```python
from build123d import *

# Parameters (mm, degrees)
F0_R      = 13
F5_DEPTH  = 15
F4_R      = 8
F6_DEPTH  = 15
F3_R      = 3.2
F8_DEPTH  = 4
F9_DEPTH  = 11
F10_R     = 2.05
F11_DEPTH = 15
F12_R     = 1.5
F13_DEPTH = 25
F15_R     = 3.5
F16_DEPTH = 5
F19_DEPTH = 3


with BuildPart() as f5:
    # F0 (on Top) → F5 (new body, symmetric)
    with BuildSketch(Plane.XY):
        Circle(F0_R)
    extrude(amount=F5_DEPTH, both=True)

    # F4 (on offset) → F6 (cut)
    with BuildSketch(Plane.XY.offset(-15)):
        Circle(F4_R)
    extrude(amount=F6_DEPTH, mode=Mode.SUBTRACT)

    # F3 (on offset) → F8 (cut)
    with BuildSketch(Plane.XY.offset(15)):
        with Locations((0.0063437128, 0)):
            Circle(F3_R)
    extrude(amount=-F8_DEPTH, mode=Mode.SUBTRACT)

    # F7 (on Top) → F9 (cut)
    with BuildSketch(Plane.XY):
        with BuildLine():
            Line((1.8168599408, 2.625), (-1.8433996128, 2.625))
            ThreePointArc((-1.8433996128, 2.625), (-0.013269836, -3.2022189551), (1.8168599408, 2.625))
        make_face()
    extrude(amount=F9_DEPTH, mode=Mode.SUBTRACT)

    # F10 (on Right) → F11 (cut, symmetric)
    with BuildSketch(Plane.YZ):
        with Locations((-2.5, -7.5)):
            Circle(F10_R)
    extrude(amount=F11_DEPTH, both=True, mode=Mode.SUBTRACT)

    # F12 (on Front) → F13 (cut)
    with BuildSketch(Plane.XZ):
        with Locations((0, 7)):
            Circle(F12_R)
    extrude(amount=-F13_DEPTH, mode=Mode.SUBTRACT)

    # F15 (on offset) → F16 (cut)
    with BuildSketch(Plane.YZ.offset(11)):
        with Locations((-2.5, -7.5)):
            Circle(F15_R)
    extrude(amount=F16_DEPTH, mode=Mode.SUBTRACT)

    # F18 (on offset) → F19 (cut)
    with BuildSketch(Plane.YZ.offset(-12)):
        Polygon((-5.9460342998, -5.8984858401), (-5.6099690969, -9.683596166), (-2.1639347971, -11.2851103259), (0.9460342998, -9.1015141599), (0.6099690969, -5.316403834), (-2.8360652029, -3.7148896741), align=None)
    extrude(amount=-F19_DEPTH, mode=Mode.SUBTRACT)


solid = f5.part
```
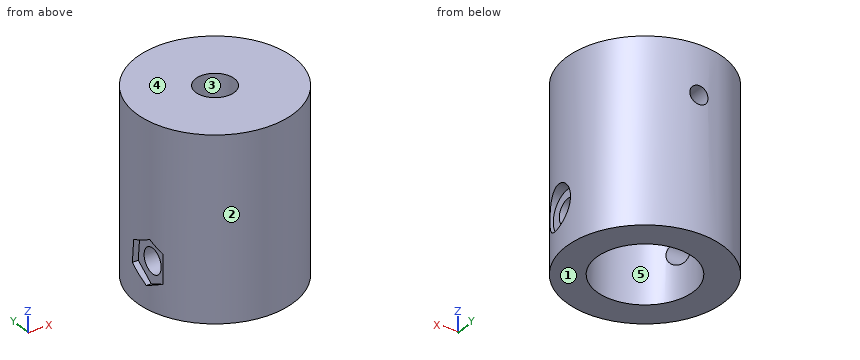
Model file for the job. Use its own axes, mm. Face numbers are marked on the shaded views. A direction names the side the tool comes from. Coordinates: 2 decimals unless noted, no trailing zeros. Order: outer loops, then holes, each group sorted by start corner. A loop starts at its lowest first (then second) coordinate and runs counter-clockwise, first axis right, second up. Notation, with made-up numbers: (58.25, -39) -> (67.25, -39) arc R20 cw to (67.25, -2) -> close; hole circle Ø6 at (50.5, 73). An arc over 180 degrees is marked (long way). Return JSON: item names as keys, results as strings.
Item 1: Pin check, flat tips, straight feed: P1, Ø6, axis at x = -4, z = 5, coming from the +Y side; P2, Ø5.5, axis at y = -2.5, z = -7.5, coming from the -X side; P3, Ø4, axis at x = 0.01, y = 0, coming from the -Z side; P4, Ø5, axis at x = 2, y = 4.5, coming from the -Z side. Stop position of each tip, or through.
Model answer:
{"P1": "stops at y = 12.96", "P2": "stops at x = -12", "P3": "passes through", "P4": "stops at z = 0"}
Item 2: Slice it at A-A (z = -7.5). Write the cut outline in (x, y).
Model answer:
{"outline": "(-12.98, 0.8) -> (-12, 0.8) -> (-12, -0.45) -> (-7.99, -0.45) arc R8 cw (long way) to (7.99, -0.45) -> (11, -0.45) -> (11, 1) -> (12.96, 1) arc R13 ccw to start; (-12, -5) arc R13 ccw to (11.53, -6) -> (11, -6) -> (11, -4.55) -> (6.58, -4.55) arc R8 cw to (-6.58, -4.55) -> (-12, -4.55) -> close"}
Item 3: 3-axis set-ups, long thin cutter, end or side, ignore diameter. For the marked faces 4 and 5: which of +Z, -Z, +X, -X, +Y, -Y reach the whole face in a straight line?
Model answer:
{"face 4": "+Z, +X, -X, +Y, -Y", "face 5": "-Z"}
Item 4: Mould opens along Y. For the marked faces 1, 2 and 3 say: pulls with the +Y half, pulls with the -Y half, needs draft (parallel to the pull), parting line crosses it, or undercut.
Model answer:
{"face 1": "needs draft", "face 2": "parting line crosses it", "face 3": "undercut"}
Item 5: Slice it at C-C (x = -9.25). Write the cut outline in (y, z).
Model answer:
{"outline": "(-9.13, -15) -> (9.13, -15) -> (9.13, 15) -> (-9.13, 15) -> close; hole circle Ø4.1 at (-2.5, -7.5)"}
Item 6: Slice it at D-D (z = 10.5). Write the cut outline in (x, y) (3 decimals).
Model answer:
{"outline": "circle Ø26 at (0, 0); hole (-1.843, 2.625) arc R3.201 ccw (long way) to (1.817, 2.625) -> close"}
Item 7: Wall check: line 1 along X through (y, z) = (0, 12.6); line 2 along X through (y, z) = (0.25, -6); line 3 along Z through (x, y) = (8.2, -2.5). Give the ranges that are in metal, low to high. Write a range as from..to.
Model answer:
{"line 1": "x = -13..-3.19, 3.21..13", "line 2": "x = -12..-8, 8..11", "line 3": "z = -15..-9.55, -5.45..15"}
Item 8: Slice it at B-B (y = 4.75). Write the cut outline in (x, z), then the cut area to 3 significant figures.
Model answer:
{"outline": "(-12.1, -15) -> (-6.44, -15) -> (-6.44, 0) -> (6.44, 0) -> (6.44, -15) -> (12.1, -15) -> (12.1, 15) -> (-12.1, 15) -> close; hole circle Ø3 at (0, 7)", "area": "526 mm²"}
